from build123d import *

# Parameters (mm, degrees)
SKETCH3_W           = 139.7
SKETCH3_H           = 88.9
BOSS_EXTRUDE2_DEPTH = 43.18
CUT_EXTRUDE1_DEPTH  = 83.82
CUT_EXTRUDE2_DEPTH  = 94.377392339
CHAMFER1_SIZE       = 5.08
FILLET1_R           = 1.27
FILLET2_R           = 6.35
FILLET3_R           = 2.54
FILLET4_R           = 1.27


with BuildPart() as part:
    # Sketch3 → Boss-Extrude2 (new body)
    with BuildSketch(Plane(origin=(0, 0, 0), x_dir=(1, 0, 0), z_dir=(0, 1, 0))):
        Rectangle(SKETCH3_W, SKETCH3_H)
    extrude(amount=BOSS_EXTRUDE2_DEPTH)

    # Sketch4 → Cut-Extrude1 (cut)
    with BuildSketch(Plane.XY.offset(44.45)):
        Polygon((-57.15, 43.18), (57.15, 43.18), (47.214435647, 21.873113486), (21.814435647, 21.873113486), (15.24, 3.81), (-15.24, 3.81), (-21.814435647, 21.873113486), (-47.214435647, 21.873113486), align=None)
    extrude(amount=-CUT_EXTRUDE1_DEPTH, mode=Mode.SUBTRACT)

    # Sketch6 → Cut-Extrude2 (cut, through all)
    with BuildSketch(Plane(origin=(0, 43.18, 0), x_dir=(1, 0, 0), z_dir=(0, 1, 0))):
        with BuildLine():
            Line((-6.35, -19.05), (-6.35, 19.05))
            ThreePointArc((-6.35, 19.05), (0, 25.4), (6.35, 19.05))
            Line((6.35, 19.05), (6.35, -19.05))
            ThreePointArc((6.35, -19.05), (0, -25.4), (-6.35, -19.05))
        make_face()
    extrude(amount=-CUT_EXTRUDE2_DEPTH, mode=Mode.SUBTRACT)

    # Chamfer1
    chamfer1_edges = [part.edges().sort_by_distance(p)[0] for p in [
        (69.85, 21.59, 44.45),
        (-69.85, 21.59, 44.45),
        (-69.85, 21.59, -44.45),
        (69.85, 21.59, -44.45),
    ]]
    chamfer(chamfer1_edges, length=CHAMFER1_SIZE)

    # Fillet1
    fillet1_edges = [part.edges().sort_by_distance(p)[0] for p in [
        (-69.85, 43.18, 0),
        (69.85, 43.18, 0),
    ]]
    fillet(fillet1_edges, radius=FILLET1_R)

    # Fillet2
    fillet2_edges = [part.edges().sort_by_distance(p)[0] for p in [
        (-47.214435647, 21.873113486, 2.54),
        (47.214435647, 21.873113486, 2.54),
        (21.814435647, 21.873113486, 2.54),
        (15.24, 3.81, 2.54),
        (-15.24, 3.81, 2.54),
        (-21.814435647, 21.873113486, 2.54),
    ]]
    fillet(fillet2_edges, radius=FILLET2_R)

    # Fillet3
    fillet3_edges = [part.edges().sort_by_distance(p)[0] for p in [
        (53.037046969, 34.359743762, -39.37),
        (34.714896503, 21.873113486, -39.37),
        (-34.714896503, 21.873113486, -39.37),
        (-18.527217824, 12.841556743, -39.37),
        (0, 3.81, -39.37),
        (18.527217824, 12.841556743, -39.37),
        (-46.580892004, 22.867577805, -39.37),
        (-14.435892503, 4.958384519, -39.37),
        (14.435892503, 4.958384519, -39.37),
        (46.580892004, 22.867577805, -39.37),
        (22.618543144, 20.724728967, -39.37),
        (-22.618543144, 20.724728967, -39.37),
        (-53.037046969, 34.359743762, -39.37),
    ]]
    fillet(fillet3_edges, radius=FILLET3_R)

    # Fillet4
    fillet4_edges = [part.edges().sort_by_distance(p)[0] for p in [
        (6.35, 3.81, 0),
        (0, 3.81, -25.4),
        (-6.35, 3.81, 0),
        (0, 3.81, 25.4),
    ]]
    fillet(fillet4_edges, radius=FILLET4_R)


solid = part.part
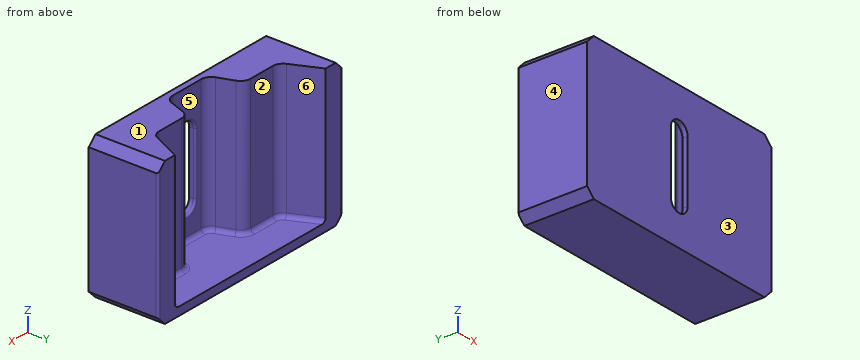
Read the model definition and answer for the solid it produces. Units are mm, in the model's axes. Face numbers are marked on the shaded views. A direction names the side the tool comes from. Round coordinates to 2 decimals unless told otherwise and drop trailing zeros. Order: outer loops, then holes, each group sorted by start corner. A loop starts at its lowest first (then second) coordinate and runs counter-clockwise, first axis right, second up.
1) The part is cut by section A-A on x = 0. Write down the section's boundary in (y, z), plus the area to 3 significant figures.
2) The mould has two halves that part along X. Classify the marked faces 3, 4, 5 and 6: released by +X, released by -X, zero draft, split by the parting line, or undercut.
3) For the marked faces 1 and 2, determine the directions among +Z, -Z, +X, -X, +Y, -Y from which every point of the face is accessible in a straight line to the end or side of a thin tool.
4) Straight lines are drawn through the part: L1, parallel to X at y = 2.5, z = -5.5; L2, parallel to Z at x = 10.5, y = 27; L3, parallel to X at y = 18.5, z = -7. For each, find the intervals that lie inside material, in ascending order.
5) The part is cut by section B-B on z = 13. Write down the section's boundary in (x, y), plus the area to 3 significant figures.
6) The part is cut by section C-C on z = 33. Write down the section's boundary in (x, y).
7) Flat-ended cylindrical pins translate along their axes: pin 1 (3 mm diameter, centred on x = 17, y = 34, fed in from +Z); pin 2 (18.5 mm diameter, centred on x = -31, z = 15.5, fed in from +Y); pin 3 (6 mm diameter, centred on x = -19, z = 2.5, fed in from +Y). Find the tip coordinate at first contact, or state that the pin passes through.
Resolved:
1. outline: (0, -44.45) - (43.18, -44.45) - (43.18, -39.37) - (6.35, -39.37) arc R2.54 cw to (3.81, -36.83) - (3.81, -26.67) arc R1.27 ccw to (2.54, -25.4) - (0, -25.4) - close; (0, 25.4) - (2.54, 25.4) arc R1.27 ccw to (3.81, 26.67) - (3.81, 44.45) - (0, 44.45) - close
1. area: 346 mm2
2. face 3: zero draft
2. face 4: released by -X
2. face 5: undercut
2. face 6: undercut
3. face 1: +Z, +X, -X, +Y, -Y
3. face 2: +Z, +Y
4. L1: x = -69.85 to -6.35, 6.35 to 69.85
4. L2: z = -44.45 to -39.37
4. L3: x = -69.85 to -20.65, 20.65 to 69.85
5. outline: (-69.85, 0) - (-6.35, 0) - (-6.35, 2.54) arc R1.27 ccw to (-7.62, 3.81) - (-10.79, 3.81) arc R6.35 cw to (-16.76, 7.99) - (-20.29, 17.69) arc R6.35 ccw to (-26.26, 21.87) - (-43.17, 21.87) arc R6.35 cw to (-48.92, 25.54) - (-57.15, 43.18) - (-68.58, 43.18) arc R1.27 ccw to (-69.85, 41.91) - close; (6.35, 0) - (69.85, 0) - (69.85, 41.91) arc R1.27 ccw to (68.58, 43.18) - (57.15, 43.18) - (48.92, 25.54) arc R6.35 cw to (43.17, 21.87) - (26.26, 21.87) arc R6.35 ccw to (20.29, 17.69) - (16.76, 7.99) arc R6.35 cw to (10.79, 3.81) - (7.62, 3.81) arc R1.27 ccw to (6.35, 2.54) - close
5. area: 3,100 mm2
6. outline: (-69.85, 0) - (69.85, 0) - (69.85, 41.91) arc R1.27 ccw to (68.58, 43.18) - (57.15, 43.18) - (48.92, 25.54) arc R6.35 cw to (43.17, 21.87) - (26.26, 21.87) arc R6.35 ccw to (20.29, 17.69) - (16.76, 7.99) arc R6.35 cw to (10.79, 3.81) - (-10.79, 3.81) arc R6.35 cw to (-16.76, 7.99) - (-20.29, 17.69) arc R6.35 ccw to (-26.26, 21.87) - (-43.17, 21.87) arc R6.35 cw to (-48.92, 25.54) - (-57.15, 43.18) - (-68.58, 43.18) arc R1.27 ccw to (-69.85, 41.91) - close
7. pin 1: stops at z = -39.37
7. pin 2: stops at y = 21.87
7. pin 3: stops at y = 20.23
